Source: three-view drawing plus pictorial views. Frame: mm from the lowest corner of the part. Give positions to 0.01 mm unless a question says otherwise; leave off trailing zeros. Order: outer loops, then holes, each group sorted by start corner. A loop starts at its lowest first (then second) coordinate and runs counter-clockwise, first axis right, second up.
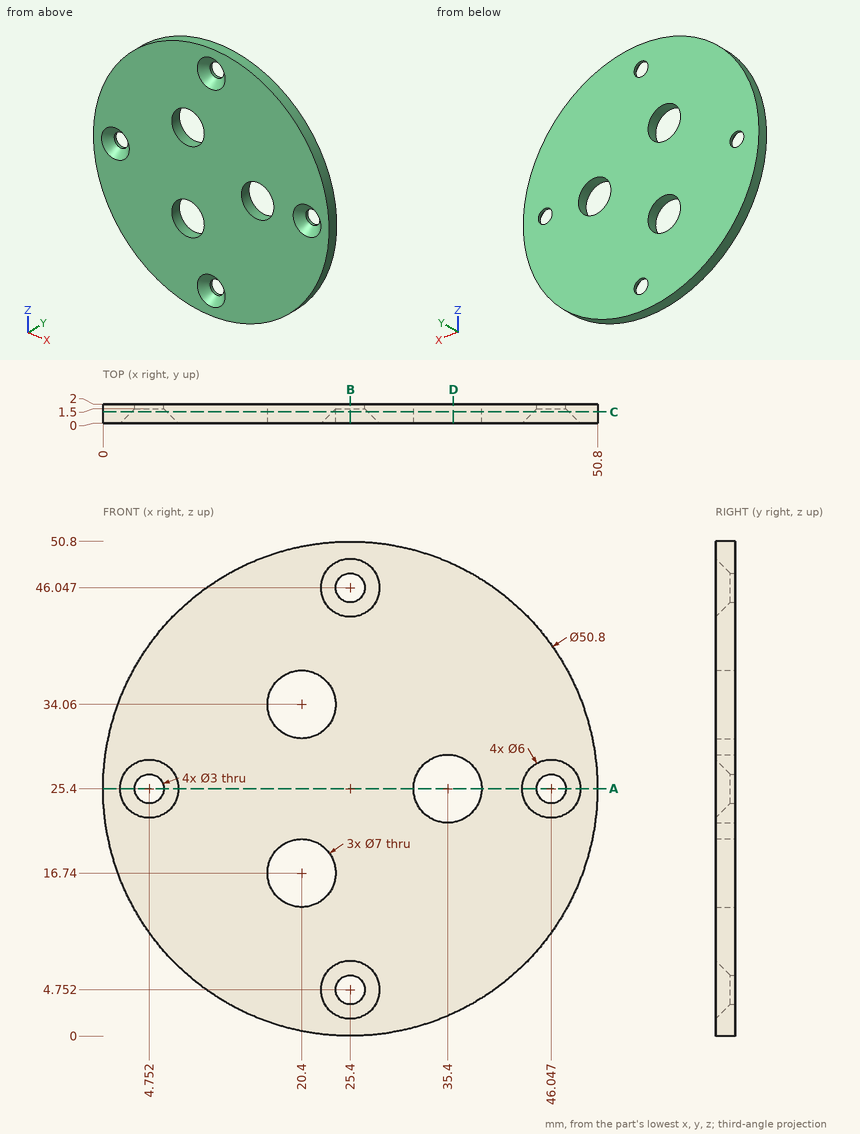
1) Section query A-A on z = 25.4. Output: boundary loops of the cut face in (x, y).
Checks:
outline: (0, 0) - (1.75, 0) - (3.25, 1.5) - (3.25, 2) - (0, 2) - close; (6.25, 1.5) - (7.75, 0) - (31.9, 0) - (31.9, 2) - (6.25, 2) - close; (38.9, 0) - (43.05, 0) - (44.55, 1.5) - (44.55, 2) - (38.9, 2) - close; (47.55, 1.5) - (49.05, 0) - (50.8, 0) - (50.8, 2) - (47.55, 2) - close
2) Ray query, L1, parallel to Z at x = 20.4, y = 0.5; L2, parallel to Z at x = 3.5, y = 1.4 (1 decimal); L3, parallel to Z at x = 19, y = 0.6. Return the intervals inside material, ascending.
Checks:
L1: z = 0.5 to 13.24, 20.24 to 30.56, 37.56 to 50.3
L2: z = 12.5 to 24.4, 26.4 to 38.3
L3: z = 0.82 to 13.53, 19.95 to 30.85, 37.27 to 49.98
3) Section query B-B on x = 25.4. Output: boundary loops of the cut face in (y, z).
Checks:
outline: (0, 0) - (2, 0) - (2, 3.25) - (1.5, 3.25) - (0, 1.75) - close; (0, 7.75) - (1.5, 6.25) - (2, 6.25) - (2, 44.55) - (1.5, 44.55) - (0, 43.05) - close; (0, 49.05) - (1.5, 47.55) - (2, 47.55) - (2, 50.8) - (0, 50.8) - close
4) Section query C-C on y = 1.2. Output: boundary loops of the cut face in (x, z), and give its area (3 significant figures).
Checks:
outline: circle Ø50.8 at (25.4, 25.4); hole circle Ø3.6 at (4.75, 25.4); hole circle Ø7 at (20.4, 16.74); hole circle Ø7 at (20.4, 34.06); hole circle Ø3.6 at (25.4, 4.75); hole circle Ø3.6 at (25.4, 46.05); hole circle Ø7 at (35.4, 25.4); hole circle Ø3.6 at (46.05, 25.4)
area: 1,870 mm2
5) Section query D-D on x = 36. Output: boundary loops of the cut face in (y, z).
Checks:
outline: (0, 2.32) - (2, 2.32) - (2, 21.95) - (0, 21.95) - close; (0, 28.85) - (2, 28.85) - (2, 48.48) - (0, 48.48) - close
6) First-contact query: pin 1 Ø10 at (x, z) = (37.5, 9.5) entering from -Y. Flat tip, straight axial feed; report the tip coordinate or a pass-through.
Checks:
pin 1: stops at y = 0
